Autodesk Inventor part; units mm, degrees
ref_plane "YZ Plane" through (0, 0, 0) normal (1, 0, 0) x (0, 1, 0)
ref_plane "XZ Plane" through (0, 0, 0) normal (0, 1, 0) x (-1, 0, 0)
ref_plane "XY Plane" through (0, 0, 0) normal (0, 0, 1) x (1, 0, 0)
sketch "スケッチ1" plane through (0, 0, 0) normal (0, 0, 1) x (1, 0, 0)
  circle A0 centre (0, 0) radius 19
  line L0 (-19, 19) -> (19, 19)
  line L1 (19, 19) -> (19, -19)
  line L2 (19, -19) -> (-19, -19)
  line L3 (-19, -19) -> (-19, 19)
  dimension "d0" = 38
extrude "押し出し1" add sketch "スケッチ1" along normal blind 3
sketch "スケッチ2" plane through (0, 0, 3) normal (0, 0, 1) x (1, 0, 0)
  circle A0 centre (0, 0) radius 7
  dimension "d3" = 14
extrude "押し出し2" cut sketch "スケッチ2" against normal blind 3
sketch "スケッチ3" plane through (0, 0, 3) normal (0, 0, 1) x (1, 0, 0)
  circle A0 centre (0, 0) radius 19
  line L0 (0, 0) -> (-13.435, 13.435)
  line L1 (0, 0) -> (0, 19)
  point P0 (-13.435, -13.435)
  point P1 (13.435, -13.435)
  point P2 (13.435, 13.435)
  dimension "d6" = 38
  dimension "d7" = 45
  dimension "d10" = 360
hole "穴1" at (-13.435, 13.435, 3) at (-13.435, -13.435, 3) at (13.435, -13.435, 3) at (13.435, 13.435, 3) direction (0, 0, -1) diameter 3.2 end through all
fillet "フィレット1" radius 10 4 edges at (-19, 19, 1.5) (19, 19, 1.5) (19, -19, 1.5) (-19, -19, 1.5)
properties part number "hand1_part3" material "アルミニウム 6061"
For this review, take the finished solid that the model builds, in its own axes (mm). Coordinates: 2 decimals unless noted, no trailing zeros. Write each loop counter-clockwise with the first axis right and the second up, starting at its lowest first coordinate (ties: lowest second). Pieces come first, ordered by that corner, then holes. Notation, with made-up numbers: (43.25, -31) - (80.25, -31) arc R35 cw to (80.25, 1) - close; hole circle Ø9 at (82, 86.25). An arc over 180 degrees is marked (long way). Answer in a Markdown table with one row per item. Add a question column.
Q1. For probe 1 along X at (y, z) = (13, 2.6); probe 2 along Y at (x, z) = (13.5, 1.7); probe 3 along Y at (x, z) = (14, 2.5), list the stretches that pass through material, from the lowest coordinate up.
Q2. We need section A-A, the plane y = 0. State the section outline as (x, z) points.
Q3. We need section C-C, the plane z = 1.7. State the section outline as (x, y) points (3 decimals), and give its area (3 significant figures).
Q4. We need section D-D, the plane x = 14. State the section outline as (y, z) points, and give its area (3 significant figures).
Q5. Draft analysis for pull direction Y (two halves, no side actions). For faces 1 (the cylindrical face through (-16.15, -15.99, 1.52)), 2 (the cylindrical face through (-12.461, -12.165, 1.479)), 3 (the cylindrical face through (16.15, 15.99, 1.52)), 4 (the cylindrical face through (-12.016, 12.697, 1.479)), state which applies: +Y half, -Y half, draft (parallel to the pull), parting line (faces both ways), or undercut.
Q6. For P1, Ø1.5, axis at x = -12, z = 2.5, coming from the +Y side, flat-tipped, find the tip position at first contact; note if it passes through.
Answer list:
| question | item | result |
|---|---|---|
| 1 | probe 1 | x = -18.17 to -14.97, -11.9 to 11.9, 14.97 to 18.17 |
| 1 | probe 2 | y = -17.93 to -15.03, -11.84 to 11.84, 15.03 to 17.93 |
| 1 | probe 3 | y = -17.66 to -14.93, -11.94 to 11.94, 14.93 to 17.66 |
| 2 | outline | (-19, 0) - (-7, 0) - (-7, 3) - (-19, 3) - close; (7, 0) - (19, 0) - (19, 3) - (7, 3) - close |
| 3 | outline | (-19, -9) arc R10 ccw to (-9, -19) - (9, -19) arc R10 ccw to (19, -9) - (19, 9) arc R10 ccw to (9, 19) - (-9, 19) arc R10 ccw to (-19, 9) - close; hole circle Ø3.2 at (-13.435, -13.435); hole circle Ø3.2 at (-13.435, 13.435); hole circle Ø14 at (0, 0); hole circle Ø3.2 at (13.435, -13.435); hole circle Ø3.2 at (13.435, 13.435) |
| 3 | area | 1,170 mm2 |
| 4 | outline | (-17.66, 0) - (-14.93, 0) - (-14.93, 3) - (-17.66, 3) - close; (-11.94, 0) - (11.94, 0) - (11.94, 3) - (-11.94, 3) - close; (14.93, 0) - (17.66, 0) - (17.66, 3) - (14.93, 3) - close |
| 4 | area | 88.0 mm2 |
| 5 | face 1 | -Y half |
| 5 | face 2 | undercut |
| 5 | face 3 | +Y half |
| 5 | face 4 | undercut |
| 6 | P1 | stops at y = 18.74 |
